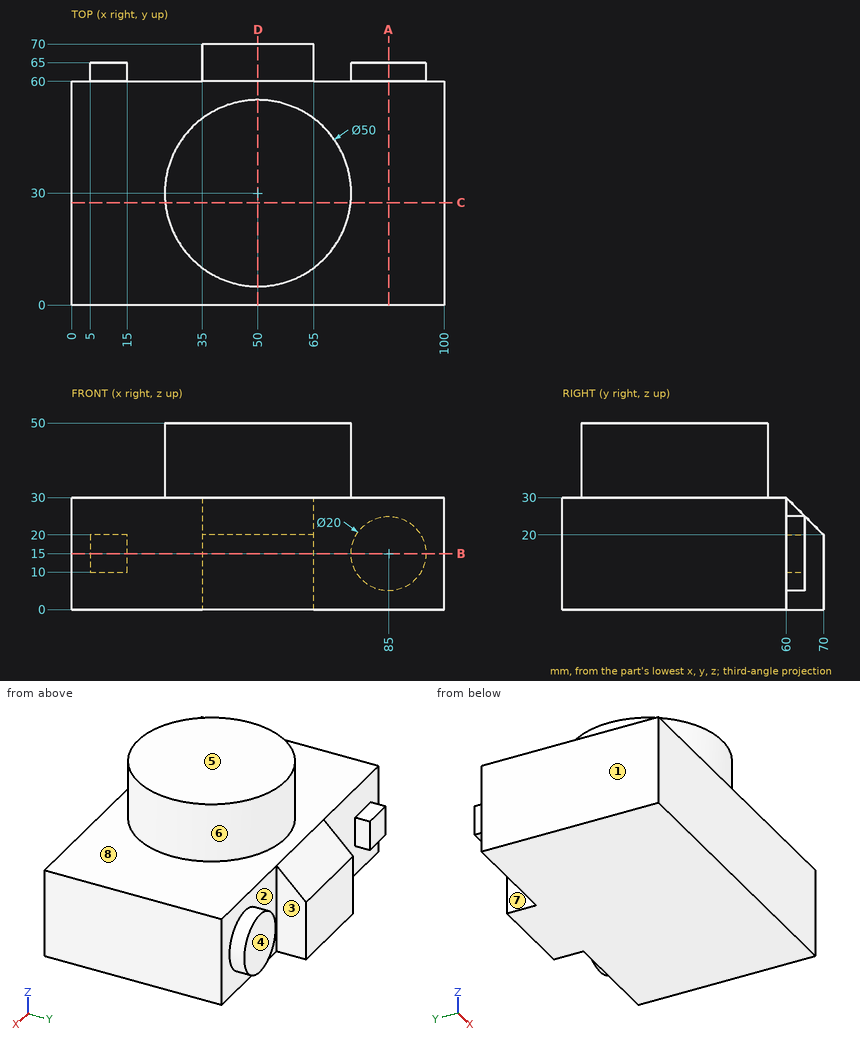
Design review of the part shown in the three views and the two pictorial views. Dimensions are in mm from the part's minimum x, y and z. A direction names the side the tool comes from. Give positions to 0.01 mm unless a question says otherwise; leave off trailing zeros. Loops run counter-clockwise (first coordinate to the right, second up) from the corner with the lowest first, then second, coordinate; pieces in that order, holes last. Notation, with made-up numbers: (79, -9.75) -> (124, -9.75) arc R20 cw to (124, 29.25) -> close; hole circle Ø11 at (56, 38.25). An arc over 180 degrees is marked (long way). Put each result on its own line as item: value. Start each with the question number.
1. For the marked faces 1, 2, 3, 4 and 5, list the 3-axis set-ups (+Z, -Z, +X, -X, +Y, -Y) from which the entire face can be reached by the end or side of a thin tool; tool diameter is ignored.
2. We need section D-D on x = 50. State the section outline as (y, z) points.
3. We need section A-A on x = 85. State the section outline as (y, z) points, then the cut area to 3 significant figures.
4. We need section C-C on y = 27.5. State the section outline as (x, z) points, then the cut area to 3 significant figures.
5. Mouldability with a two-part tool opening along X and no side actions: class the marked faces 6, 7 and 8 as released by +X, released by -X, zero draft, split by the parting line, or undercut.
6. We need section B-B on z = 15. State the section outline as (x, y) points, then the cut area to 3 significant figures.
7. Clearance check with flat-ended pins moving along their axes: P1, Ø5, axis at y = 66, z = 21, coming from the +X side; P2, Ø2.5, axis at y = 63, z = 13.5, coming from the -X side; P3, Ø3, axis at x = 23.5, z = 23, coming from the +Y side. State where each tip first meets the part, or that it passes through.
8. Wall thickness on probe 1 along Z at (x, y) = (82.5, 52.5); probe 2 along Y at (x, z) = (29, 11); probe 3 along Y at (x, z) = (38.5, 29): over which ranges is each line inside the solid? List them lowest first.
Determined:
1. face 1: +Z, -Z, -X, +Y, -Y
1. face 2: +Y
1. face 3: +Z, -Z, +Y
1. face 4: +Z, -Z, +X, +Y
1. face 5: +Z, +X, -X, +Y, -Y
2. outline: (0, 0) -> (70, 0) -> (70, 20) -> (60, 30) -> (55, 30) -> (55, 50) -> (5, 50) -> (5, 30) -> (0, 30) -> close
3. outline: (0, 0) -> (60, 0) -> (60, 5) -> (65, 5) -> (65, 25) -> (60, 25) -> (60, 30) -> (0, 30) -> close
3. area: 1,900 mm^2
4. outline: (0, 0) -> (100, 0) -> (100, 30) -> (74.87, 30) -> (74.87, 50) -> (25.13, 50) -> (25.13, 30) -> (0, 30) -> close
4. area: 3,990 mm^2
5. face 6: split by the parting line
5. face 7: undercut
5. face 8: zero draft
6. outline: (0, 0) -> (100, 0) -> (100, 60) -> (95, 60) -> (95, 65) -> (75, 65) -> (75, 60) -> (65, 60) -> (65, 70) -> (35, 70) -> (35, 60) -> (15, 60) -> (15, 65) -> (5, 65) -> (5, 60) -> (0, 60) -> close
6. area: 6,450 mm^2
7. P1: x = 94.29
7. P2: x = 5
7. P3: y = 60
8. probe 1: 0 to 30
8. probe 2: 0 to 60
8. probe 3: 0 to 61
